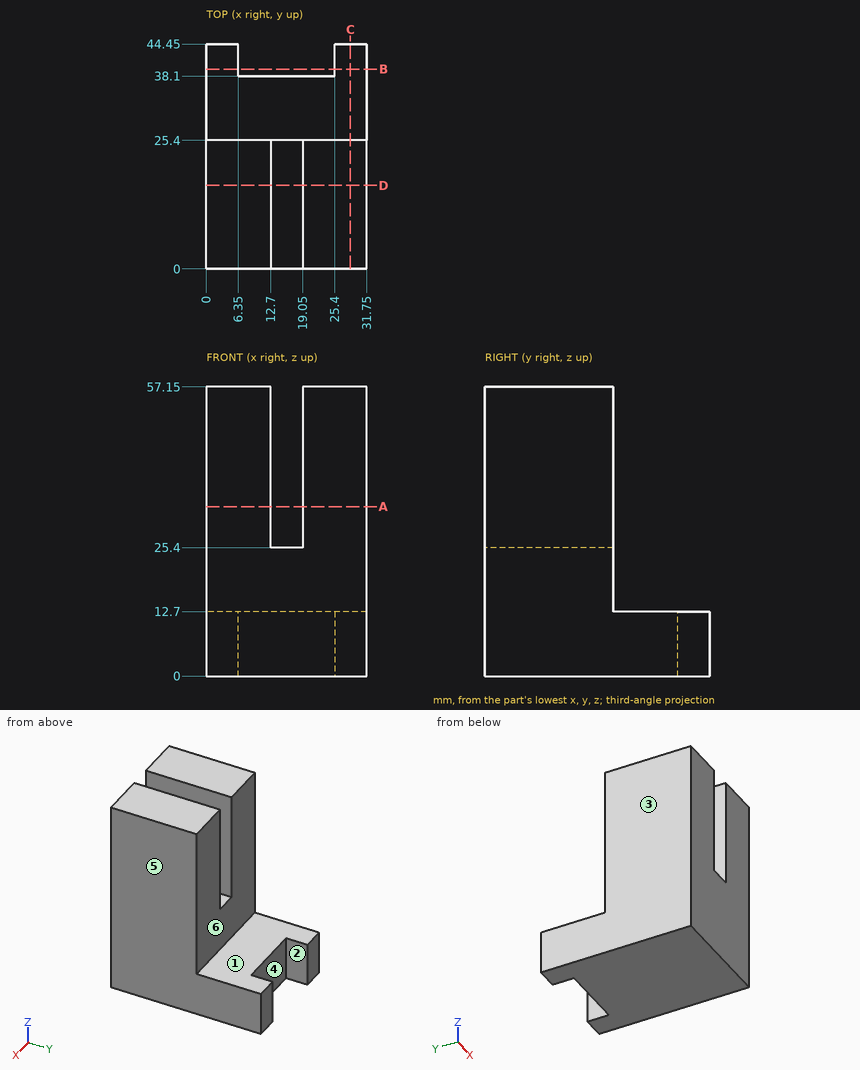
Study the drawing (mm; zero at the part's minimum x, y, z) and answer. A direction names the side the tool comes from. Round coordinates to 2 decimals unless told otherwise and drop trailing zeros. Write each loop counter-clockwise with the first axis right and the second up, starting at its lowest first coordinate (ties: lowest second). Pieces come first, ordered by that corner, then holes.
Q1. Flat-ended cylindrical pins translate along their axes: P1, Ø7, axis at x = 16, y = 10, coming from the +Z side; P2, Ø8, axis at y = 33, z = 39, coming from the +X side; P3, Ø5, axis at x = 4, z = 32.5, coming from the +Y side; P4, Ø1, axis at x = 24, y = 33.5, coming from the +Z side. Find the tip coordinate at first contact, or state that the pin passes through.
Values:
P1: stops at z = 57.15
P2: passes through
P3: stops at y = 25.4
P4: stops at z = 12.7
Q2. Find section A-A on z = 33.5. Determine the outline of the cut face in (x, y).
Values:
outline: (0, 0) - (12.7, 0) - (12.7, 25.4) - (0, 25.4) - close; (19.05, 0) - (31.75, 0) - (31.75, 25.4) - (19.05, 25.4) - close
Q3. Find section C-C on x = 28.5. Determine the outline of the cut face in (y, z).
Values:
outline: (0, 0) - (44.45, 0) - (44.45, 12.7) - (25.4, 12.7) - (25.4, 57.15) - (0, 57.15) - close
Q4. Straight lines are drawn through the part: line 1 (X direction, y = 21.5, z = 48.5); line 2 (Y direction, x = 10, z = 3.5); line 3 (Y direction, x = 20, z = 40). For each, find the intervals that lie inside material, in ascending order.
Values:
line 1: x = 0 to 12.7, 19.05 to 31.75
line 2: y = 0 to 38.1
line 3: y = 0 to 25.4
Q5. Find section B-B on y = 39.5. Determine the outline of the cut face in (x, z).
Values:
outline: (0, 0) - (6.35, 0) - (6.35, 12.7) - (0, 12.7) - close; (25.4, 0) - (31.75, 0) - (31.75, 12.7) - (25.4, 12.7) - close
Q6. The mould has two halves that part along X. Classify the marked faces 4, 5 and 6: released by +X, released by -X, zero draft, split by the parting line, or undercut.
Values:
face 4: undercut
face 5: released by +X
face 6: zero draft
Q7. Find section D-D on y = 16.5. Determine the outline of the cut face in (x, z).
Values:
outline: (0, 0) - (31.75, 0) - (31.75, 57.15) - (19.05, 57.15) - (19.05, 25.4) - (12.7, 25.4) - (12.7, 57.15) - (0, 57.15) - close
Q8. A tool of negligible diameter and unlimited length cuts with its end or side. For the marked faces 1, 2 and 3, from which of +Z, -Z, +X, -X, +Y, -Y can it reach the whole face along a straight path? Write none if from no direction.
Values:
face 1: +Z, +X, -X, +Y
face 2: +Z, -Z, +Y
face 3: +Z, -Z, -X, +Y, -Y
